Solid Edge part; units mm, degrees
sketch "Sketch1" plane through (0, 0, 0) normal (0, -1, 0) x (1, 0, 0)
  line L0 (1.5, 0) -> (3, 1.5)
  line L1 (3, 1.5) -> (3, 1.7)
  line L2 (3, 1.7) -> (0, 1.7)
  line L3 (0, 1.7) -> (0, -8.3)
  line L4 (0, -8.3) -> (1.1935, -8.3)
  line L5 (1.1935, -8.3) -> (1.5, -7.9935)
  line L6 (1.5, -7.9935) -> (1.5, -1.5)
  line L7 (1.5, -1.5) -> (1.1935, -1.5)
  line L8 (1.1935, -1.5) -> (1.1935, -1.49)
  line L9 (1.1935, -1.49) -> (1.5, -1.49)
  line L10 (1.5, -1.49) -> (1.5, 0)
  dimension "D1" = 1.5
  dimension "D2" = 1.1935
revolve "RevolvedProtrusion1" add sketch "Sketch1" angle 360 about axis through (0, 0, 54) along (0, 0, -1)
sketch "Sketch2" plane through (0, 0, 0) normal (0, -1, 0) x (1, 0, 0)
  arc A0 (-1, 0.5) -> (0, 0) centre (0, 1.25) ccw
  line L0 (0, 0.5) -> (0, 0)
  line L1 (-1, 0.5) -> (0, 0.5)
revolve "RevolvedCutout1" cut sketch "Sketch2" angle 360 about axis through (0, 0, 54) along (0, 0, -1)
sketch "Sketch3" plane through (0, 0, 1.7) normal (0, 0, 1) x (0, -1, 0)
  line L0 (-1.1547, 0) -> (-0.5774, 1)
  line L1 (-0.5774, 1) -> (0.5774, 1)
  line L2 (0.5774, 1) -> (1.1547, 0)
  line L3 (1.1547, 0) -> (0.5774, -1)
  line L4 (0.5774, -1) -> (-0.5774, -1)
  line L5 (-0.5774, -1) -> (-1.1547, 0)
extrude "Cutout1" cut sketch "Sketch3" against normal blind 1.2
cosmetic_thread "Thread1"
sketch "Sketch4" plane through (0, 0, 0) normal (1, 0, 0) x (0, 1, 0)
  line L0 (-1.15, 1.7) -> (0, 1.036)
revolve "RevolvedCutout2" cut sketch "Sketch4" angle 360 about axis through (0, 0, -57) along (0, 0, 1) material side at (0, -0.55, 1.4113)
fillet "Round1" radius 0.1 1 edges at (-1.5, 0, 0)
properties material "Stahl"
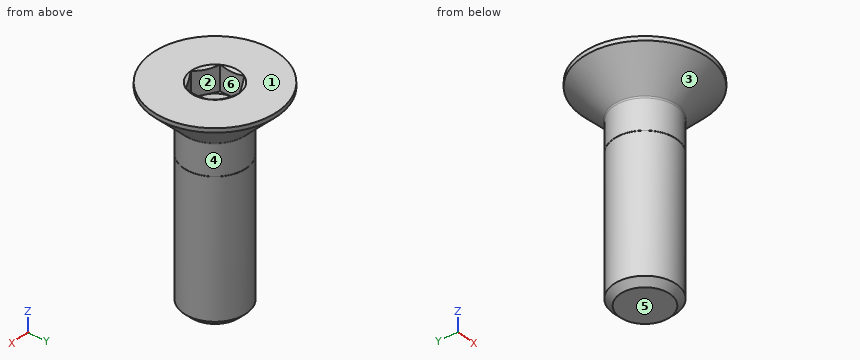
Build history of the part. All positions in model axes, mm. Face numbers are marked on the shaded views. A direction names the side the tool comes from. Give positions to 0.01 mm unless a question says otherwise; leave off trailing zeros. Loops run counter-clockwise (first coordinate to the right, second up) from the corner with the lowest first, then second, coordinate; pieces in that order, holes last. Notation, with made-up numbers: (51, 9) -> (70, 9) arc R20 cw to (70, 38) -> close; hole circle Ø7 at (39.5, -30.5). An arc over 180 degrees is marked (long way). Answer in a Markdown table with one row per item.
Item 1: Probe line 1 along X through (y, z) = (0, -3.25); line 2 along Z through (x, y) = (1, -2.5); line 3 along Y through (x, z) = (-1.25, 0.5). List the from-to ranges inside material, lowest first. Write a range as [from, to].
Findings below:
| item | result |
|---|---|
| line 1 | x = [-1.5, 1.5] |
| line 2 | z = [1.19, 1.7] |
| line 3 | y = [-1.56, 1.56] |
Item 2: Slice it at A-A on z = -4.75. Write the cut outline in (x, y), plus the area to 3 significant figures.
Findings below:
| item | result |
|---|---|
| outline | circle Ø3 at (0, 0) |
| area | 7.07 mm² |
Item 3: Mould opens along X. For the marked faces 1, 2 and 3 say: pulls with the +X half, pulls with the -X half, needs draft (parallel to the pull), parting line crosses it, or undercut.
Findings below:
| item | result |
|---|---|
| face 1 | needs draft |
| face 2 | undercut |
| face 3 | parting line crosses it |
Item 4: Tool access for the marked faces 4, 5 and 6: list every direction of +Z, -Z, +X, -X, +Y, -Y with a clear straight run to the whole face (end or side of a thin tool).
Findings below:
| item | result |
|---|---|
| face 4 | -Z |
| face 5 | -Z, +X, -X, +Y, -Y |
| face 6 | +Z |
Item 5: Flat gauge pins, fed straight in: P1, Ø1, axis at x = 2, z = 0.5, coming from the +Y side; P2, Ø1.5, axis at x = 1, z = -6, coming from the -Y side; P3, Ø2, axis at x = 1, z = 0.5, coming from the +Y side. Where does each tip first touch, or does it go through?
Findings below:
| item | result |
|---|---|
| P1 | stops at y = 1.69 |
| P2 | stops at y = -1.48 |
| P3 | stops at y = 2.87 |
